from build123d import *

# Parameters (mm, degrees)
F0_W     = 20
F0_H     = 15
F1_DEPTH = 25


with BuildPart() as f1:
    # F0 (on Top) → F1 (new body)
    with BuildSketch(Plane.XY):
        Polygon((-6.619532, 52.380648), (-6.624972, -32.619352), (13.375028, -32.619352), align=None)
        with Locations((3.375028, -40.119352)):
            Rectangle(F0_W, F0_H)
        Polygon((-6.624972, -47.619352), (-6.624972, -32.619352), (-16.624971, -47.622049), align=None)
        Polygon((23.375028, -47.622049), (13.375028, -32.619352), (13.375028, -47.619352), align=None)
    extrude(amount=-F1_DEPTH)


solid = f1.part
Verification items for the finished model (mm, model axes). Coordinates: 2 decimals unless noted, no trailing zeros. Order: outer loops, then holes, each group sorted by start corner. A loop starts at its lowest first (then second) coordinate and runs counter-clockwise, first axis right, second up. Notation, with made-up numbers: M -13,42 L 32,42 A16 ccw 32,52 Z; hole C 44,80.5 d5. An arc over 180 degrees is marked long. Write each question's results on one line, items separated by ' | '.
1) Section check C-C on x = -12. Record the cut outline in (y, z).
Solved:
outline: M -47.62,-25 L -40.68,-25 L -40.68,0 L -47.62,0 Z
2) Gauge pin test, flat ends, axial feed: pin 1 Ø4 at (x, z) = (10.5, -5) entering from -Y; pin 2 Ø2 at (y, z) = (-7, -6.5) entering from -X; pin 3 Ø1.5 at (y, z) = (4.5, -16) entering from +X. Record the tip position at first contact, or that the pin passes through.
Solved:
pin 1: stops at y = -47.62 | pin 2: stops at x = -6.62 | pin 3: stops at x = 4.82
3) Section check A-A on z = -15. Record the cut outline in (x, y).
Solved:
outline: M -16.62,-47.62 L -6.62,-47.62 L 13.38,-47.62 L 23.38,-47.62 L 13.38,-32.62 L -6.62,52.38 L -6.62,-32.62 Z
4) Section check B-B on y = 43. Record the cut outline in (x, z).
Solved:
outline: M -6.62,-25 L -4.41,-25 L -4.41,0 L -6.62,0 Z
5) Scan lines: line 1 along X through (y, z) = (-27, -0.75); line 2 along X through (y, z) = (19, -5.5); line 3 along Y through (x, z) = (19, -23). Record each from-to range of solid material in increasing order. Write a range as [from, to].
Solved:
line 1: x = [-6.62, 12.05] | line 2: x = [-6.62, 1.23] | line 3: y = [-47.62, -41.06]
